Read the model definition and answer for the solid it produces. Units are mm, in the model's axes. A direction names the side the tool comes from. Round coordinates to 2 decimals unless told otherwise and drop trailing zeros. Order: outer loops, then holes, each group sorted by start corner. A loop starts at its lowest first (then second) coordinate and runs counter-clockwise, first axis right, second up.
from build123d import *

# Parameters (mm, degrees)
BOSS_EXTRUDE1_DEPTH = 7
SKETCH2_R           = 1.35
CUT_EXTRUDE1_DEPTH  = 1.7
SKETCH3_R           = 10
BOSS_EXTRUDE2_DEPTH = 2
SKETCH4_R           = 5.6
BOSS_EXTRUDE3_DEPTH = 4
SKETCH5_R           = 10
BOSS_EXTRUDE4_DEPTH = 2
SKETCH6_R           = 3.15
CUT_EXTRUDE2_DEPTH  = 17.248076809
SKETCH7_R           = 17.649258726
CUT_EXTRUDE3_DEPTH  = 7


with BuildPart() as part:
    # Sketch1 → Boss-Extrude1 (new body)
    with BuildSketch(Plane.XY):
        with BuildLine():
            Line((-5, 0), (-5, -8))
            Line((-5, -8), (5, -8))
            Line((5, -8), (5, 0))
            ThreePointArc((5, 0), (0, 5), (-5, 0))
        make_face()
        with BuildLine():
            Line((-3.5, -6.3), (-3.5, -2.3))
            Line((-3.5, -2.3), (-1.926136028, -2.3))
            ThreePointArc((-1.926136028, -2.3), (-1.269171366, 2.718309041), (3, 0))
            ThreePointArc((3, 0), (2.718309041, -1.269171366), (1.926136028, -2.3))
            Line((1.926136028, -2.3), (3.5, -2.3))
            Line((3.5, -2.3), (3.5, -6.3))
            Line((3.5, -6.3), (-3.5, -6.3))
        make_face(mode=Mode.SUBTRACT)
    extrude(amount=BOSS_EXTRUDE1_DEPTH)

    # Sketch2 → Cut-Extrude1 (cut)
    with BuildSketch(Plane.XZ.offset(8)):
        with Locations(Location((0, 4, 0), (0, 0, 270))):
            Circle(SKETCH2_R)
    extrude(amount=-CUT_EXTRUDE1_DEPTH, mode=Mode.SUBTRACT)

    # Sketch3 → Boss-Extrude2 (add)
    with BuildSketch(Plane(origin=(0, 0, 0), x_dir=(-1, 0, 0), z_dir=(0, 0, -1))):
        Circle(SKETCH3_R)
    extrude(amount=BOSS_EXTRUDE2_DEPTH)

    # Sketch4 → Boss-Extrude3 (add)
    with BuildSketch(Plane(origin=(0, 0, -2), x_dir=(-1, 0, 0), z_dir=(0, 0, -1))):
        Circle(SKETCH4_R)
    extrude(amount=BOSS_EXTRUDE3_DEPTH)

    # Sketch5 → Boss-Extrude4 (add)
    with BuildSketch(Plane(origin=(0, 0, -6), x_dir=(-1, 0, 0), z_dir=(0, 0, -1))):
        Circle(SKETCH5_R)
    extrude(amount=BOSS_EXTRUDE4_DEPTH)

    # Sketch6 → Cut-Extrude2 (cut, through all)
    with BuildSketch(Plane.XY):
        Circle(SKETCH6_R)
    extrude(amount=-CUT_EXTRUDE2_DEPTH, mode=Mode.SUBTRACT)

    # Sketch7 → Cut-Extrude3 (cut)
    with BuildSketch(Plane.XY.offset(7)):
        Circle(SKETCH7_R)
    extrude(amount=-CUT_EXTRUDE3_DEPTH, mode=Mode.SUBTRACT)


solid = part.part
Q1. A cutting plane is placed at A-A, the plane x = 6. Give the vertices of the cut face in (y, z), plus the area to 3 significant figures.
Outcome:
outline: (-8, -8) - (8, -8) - (8, -6) - (-8, -6) - close; (-8, -2) - (8, -2) - (8, 0) - (-8, 0) - close
area: 64.0 mm2
Q2. A cutting plane is placed at C-C, the plane x = 8. Give the vertices of the cut face in (y, z), plus the area to 3 significant figures.
Outcome:
outline: (-6, -8) - (6, -8) - (6, -6) - (-6, -6) - close; (-6, -2) - (6, -2) - (6, 0) - (-6, 0) - close
area: 48.0 mm2
Q3. Straight lines are drawn through the part: probe 1 along Z at (x, y) = (-3.5, 6.25); probe 2 along Y at (x, z) = (0, -2.75); probe 3 along Y at (x, z) = (-1, -0.5). For each, find the intervals that lie inside material, in ascending order.
Outcome:
probe 1: z = -8 to -6, -2 to 0
probe 2: y = -5.6 to -3.15, 3.15 to 5.6
probe 3: y = -9.95 to -2.99, 2.99 to 9.95
Q4. A cutting plane is placed at D-D, the plane z = -6.5. Give the vertices of the cut face in (x, y), plus the area to 3 significant figures.
Outcome:
outline: circle Ø20 at (0, 0); hole circle Ø6.3 at (0, 0)
area: 283 mm2
Q5. A cutting plane is placed at B-B, the plane y = 0. Give the vertices of the cut face in (x, z), plus the area to 3 significant figures.
Outcome:
outline: (-10, -8) - (-3.15, -8) - (-3.15, 0) - (-10, 0) - (-10, -2) - (-5.6, -2) - (-5.6, -6) - (-10, -6) - close; (3.15, -8) - (10, -8) - (10, -6) - (5.6, -6) - (5.6, -2) - (10, -2) - (10, 0) - (3.15, 0) - close
area: 74.4 mm2
Q6. Flat-ended cylindrical pins translate along their axes: pin 1 (8 mm diameter, centred on x = -3, y = -6.5, fed in from +Z); pin 2 (2 mm diameter, centred on y = -5.5, z = -2, fed in from +X); pin 3 (1 mm diameter, centred on y = -5.5, z = -4.5, fed in from -X). Find the tip coordinate at first contact, or state that the pin passes through.
Outcome:
pin 1: stops at z = 0
pin 2: stops at x = 8.93
pin 3: stops at x = -2.52
Q7. For faces 1 (the face through (2.17, -9.76, -0.99)), 2 (the face through (-4.3, -4.3, -6)), determine the directions among +Z, -Z, +X, -X, +Y, -Y from which every point of the face is accessible in a straight line to the end or side of a thin tool.
Outcome:
face 1: +Z, -Z
face 2: none
Q8. For a pull along Z with two mould halves and no side action, classify faces 3 (the face through (-2.4, 2.4, 0)), 4 (the face through (2.4, 2.4, -8)), 5 (the face through (5.595, 0.246, -3.972)), 6 (the face through (2.17, -9.76, -6.99)) as released by +Z, released by -Z, zero draft, split by the parting line, or undercut.
Outcome:
face 3: released by +Z
face 4: released by -Z
face 5: undercut
face 6: zero draft
